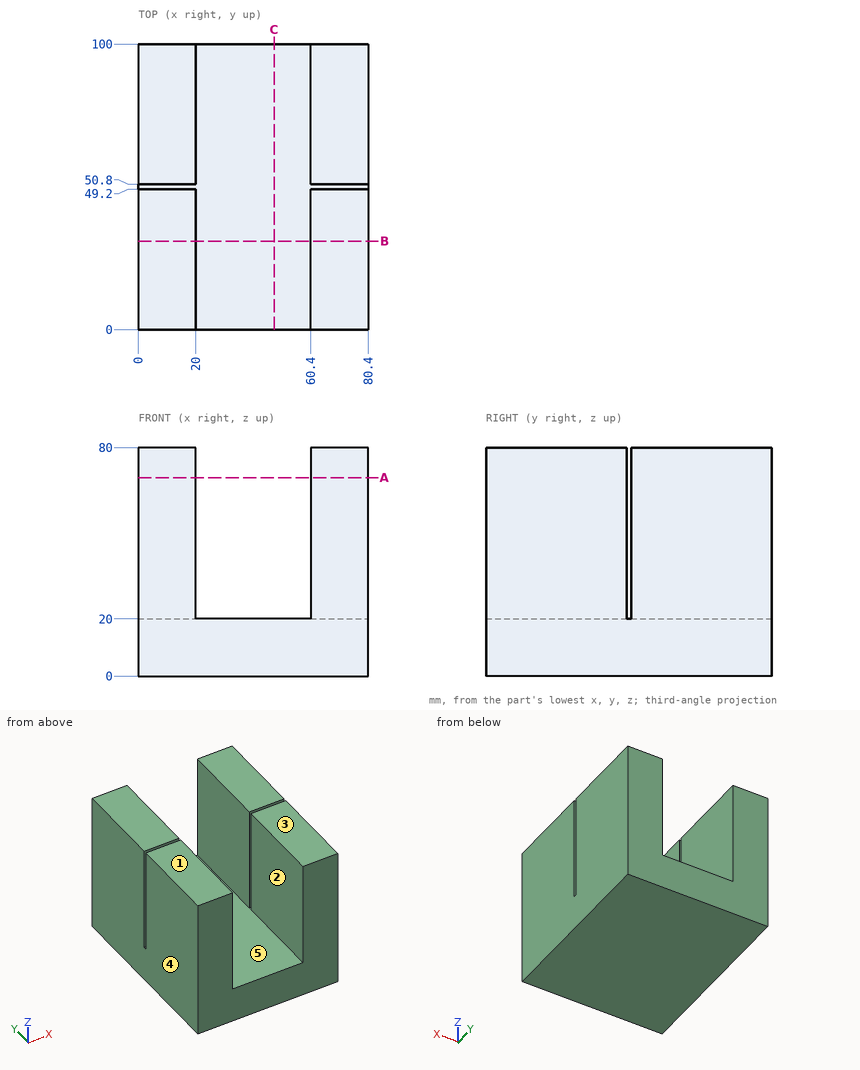
Input: dimensioned drawing with shaded views. Units: mm. Origin: part minimum x, y, z. A direction names the side the tool comes from. Round coordinates to 2 decimals unless told otherwise and drop trailing zeros. Order: outer loops, then holes, each group sorted by start corner. A loop starts at its lowest first (then second) coordinate and runs counter-clockwise, first axis right, second up. Notation, with made-up numbers: (68, 28.5) - (121, 28.5) arc R25 cw to (121, 53.5) - close; hole circle Ø3 at (65.25, -21.5). An arc over 180 degrees is marked (long way). Answer as a JSON object with one key per item and string values. Group by question number.
(1) Material intervals for probe 1 along X at (y, z) = (89, 62.5); probe 2 along Y at (x, z) = (67, 31); probe 3 along Z at (x, y) = (42.5, 83.5), sorted ascending. Write a range as from..to.
(2) Cut plane A-A (z = 69.5). Return loops of the section in (x, y).
(3) Cut plane C-C (x = 47.5). Return loops of the section in (y, z).
(4) Cut plane B-B (y = 31). Return loops of the section in (x, z).
(5) Reachability of the marked faces 1 and 2 from +Z, -Z, +X, -X, +Y, -Y: full face, straight path, thin tool, end or side. Return the list, or none.
(6) Draft query along X for the marked faces 3, 4 and 5. Return one class per face: released by +X, released by -X, zero draft, split by the parting line, or undercut.
Here are the results:
{
 "1": {"probe 1": "x = 0..20, 60.4..80.4", "probe 2": "y = 0..49.2, 50.8..100", "probe 3": "z = 0..20"},
 "2": {"outline": "(0, 0) - (20, 0) - (20, 49.2) - (0, 49.2) - close; (0, 50.8) - (20, 50.8) - (20, 100) - (0, 100) - close; (60.4, 0) - (80.4, 0) - (80.4, 49.2) - (60.4, 49.2) - close; (60.4, 50.8) - (80.4, 50.8) - (80.4, 100) - (60.4, 100) - close"},
 "3": {"outline": "(0, 0) - (100, 0) - (100, 20) - (0, 20) - close"},
 "4": {"outline": "(0, 0) - (80.4, 0) - (80.4, 80) - (60.4, 80) - (60.4, 20) - (20, 20) - (20, 80) - (0, 80) - close"},
 "5": {"face 1": "+Z, +X, -X, +Y, -Y", "face 2": "+Z, +Y, -Y"},
 "6": {"face 3": "zero draft", "face 4": "released by -X", "face 5": "undercut"}
}
